from build123d import *

# Parameters (mm, degrees)
SKETCH2_R                                       = 7.5
BOSS_EXTRUDE1_DEPTH                             = 10
CSK_FOR_M4_FLAT_HEAD_MACHINE_SCREW1_D           = 4.3
CSK_FOR_M4_FLAT_HEAD_MACHINE_SCREW1_CSINK_D     = 11.4
CSK_FOR_M4_FLAT_HEAD_MACHINE_SCREW1_CSINK_ANGLE = 90
FILLET1_R                                       = 20
V_GROOVE_CUTOUT_DEPTH                           = 3.6
STANDARD_TAPERED_INSERT_CUTOUT_DEPTH            = 59.209110795
STANDARD_TAPERED_INSERT_CUTOUT_DEPTH_BACK       = 59.209110795
SKETCH13_R                                      = 2.25
TAPER_FOR_INSERTS_SIZE                          = 0.4
TAPER_FOR_INSERTS_SIZE2                         = 1.098990968
MOVE_FACE1_BY                                   = 0.5
MOVE_FACE1_2_BY                                 = 0.5
MOVE_FACE1_3_BY                                 = 0.5
MOVE_FACE1_4_BY                                 = 0.5
MOVE_FACE1_5_BY                                 = 0.5
MOVE_FACE1_6_BY                                 = 0.5
CIRPATTERN2_COUNT                               = 3
FILLET2_R                                       = 3
SKETCH47_R                                      = 1.7
CUT_EXTRUDE1_DEPTH                              = 58.559983963
SKETCH49_W                                      = 15
SKETCH49_H                                      = 10
SKETCH49_W_2                                    = 10
SKETCH49_H_2                                    = 3
BOSS_EXTRUDE2_DEPTH                             = 40
CHAMFER1_SIZE                                   = 2
BOSS_EXTRUDE3_REACH                             = 78.74
SKETCH51_W                                      = 3
SKETCH51_H                                      = 10
BOSS_EXTRUDE4_DEPTH                             = 10
SKETCH48_R                                      = 1.7
CUT_EXTRUDE2_DEPTH                              = 93.266742447
CHAMFER4_SIZE                                   = 2
CHAMFER3_SIZE                                   = 2


with BuildPart() as part:
    # Sketch2 → Boss-Extrude1 (new body)
    with BuildSketch(Plane.XY):
        Polygon((-24.25, 45), (24.25, 45), (24.25, -5.917840259), (35.54293994, -12.437822174), (29.54293994, -22.830127019), (-29.54293994, -22.830127019), (-35.54293994, -12.437822174), (-24.25, -5.917840259), align=None)
        Circle(SKETCH2_R, mode=Mode.SUBTRACT)
    extrude(amount=BOSS_EXTRUDE1_DEPTH)

    # CSK for M4 Flat Head Machine Screw1 (through all)
    with Locations(Plane.XY.offset(10)):
        with Locations((-25.980762114, -15), (0, 30), (25.980762114, -15)):
            CounterSinkHole(CSK_FOR_M4_FLAT_HEAD_MACHINE_SCREW1_D / 2, CSK_FOR_M4_FLAT_HEAD_MACHINE_SCREW1_CSINK_D / 2, counter_sink_angle=CSK_FOR_M4_FLAT_HEAD_MACHINE_SCREW1_CSINK_ANGLE)

    # Fillet1
    fillet1_edges = [part.edges().sort_by_distance(p)[0] for p in [
        (24.25, -5.917840259, 5),
        (-24.25, -5.917840259, 5),
    ]]
    fillet(fillet1_edges, radius=FILLET1_R)

    # Sketch44 → v-groove cutout (cut)
    with BuildSketch(Plane(origin=(0, 0, 0), x_dir=(-1, 0, 0), z_dir=(0, 0, -1))):
        with BuildLine():
            Line((10.392304845, 10), (-10.392304845, 10))
            ThreePointArc((-10.392304845, 10), (-13.856406461, 8), (-13.856406461, 4))
            Line((-13.856406461, 4), (-3.464101615, -14))
            ThreePointArc((-3.464101615, -14), (0, -16), (3.464101615, -14))
            Line((3.464101615, -14), (13.856406461, 4))
            ThreePointArc((13.856406461, 4), (13.856406461, 8), (10.392304845, 10))
        make_face()
    extrude(amount=-V_GROOVE_CUTOUT_DEPTH, mode=Mode.SUBTRACT)

    # Sketch13 → standard tapered insert cutout (cut, two sides: drawn at the far end of the back side and taken through both)
    with BuildSketch(Plane(origin=(0, 0, 0), x_dir=(-1, 0, 0), z_dir=(0, 0, -1)).offset(-STANDARD_TAPERED_INSERT_CUTOUT_DEPTH_BACK)):
        with Locations((-10.392304845, 6)):
            Circle(SKETCH13_R)
        with Locations((10.392304845, 6)):
            Circle(SKETCH13_R)
        with Locations((0, -12)):
            Circle(SKETCH13_R)
    extrude(amount=STANDARD_TAPERED_INSERT_CUTOUT_DEPTH + STANDARD_TAPERED_INSERT_CUTOUT_DEPTH_BACK, mode=Mode.SUBTRACT)

    # taper for inserts
    taper_for_inserts_edges = [part.edges().sort_by_distance(p)[0] for p in [
        (12.642304845, 6, 10),
        (-8.142304845, 6, 10),
        (2.25, -12, 10),
    ]]
    taper_for_inserts_side = [part.faces().sort_by_distance(p)[0] for p in [
        (0, 10.687623267, 10),
    ]]
    chamfer(taper_for_inserts_edges, length=TAPER_FOR_INSERTS_SIZE, length2=TAPER_FOR_INSERTS_SIZE2, reference=taper_for_inserts_side[0])

    # Move Face1: a face moved inward by 0.5
    extrude(part.faces().sort_by_distance((-8.660254038, -5, 1.8))[0], amount=MOVE_FACE1_BY, dir=(-0.866025404, -0.5, 0), mode=Mode.SUBTRACT)

    # Move Face1 2: a curved face moved inward by 0.5
    add(Solid.thicken(part.faces().sort_by_distance((0, -16, 1.8))[0], -MOVE_FACE1_2_BY), mode=Mode.SUBTRACT)

    # Move Face1 3: a face moved inward by 0.5
    extrude(part.faces().sort_by_distance((8.660254038, -5, 1.8))[0], amount=MOVE_FACE1_3_BY, dir=(0.866025404, -0.5, 0), mode=Mode.SUBTRACT)

    # Move Face1 4: a curved face moved inward by 0.5
    add(Solid.thicken(part.faces().sort_by_distance((13.856406461, 8, 1.8))[0], -MOVE_FACE1_4_BY), mode=Mode.SUBTRACT)

    # Move Face1 5: a curved face moved inward by 0.5
    add(Solid.thicken(part.faces().sort_by_distance((-13.856406461, 8, 1.8))[0], -MOVE_FACE1_5_BY), mode=Mode.SUBTRACT)

    # Move Face1 6: a face moved inward by 0.5
    extrude(part.faces().sort_by_distance((0, 10, 1.8))[0], amount=MOVE_FACE1_6_BY, dir=(0, 1, 0), mode=Mode.SUBTRACT)

    # Sketch46 → tool ball cutout (revolve, cut)
    with BuildSketch(Plane(origin=(0, 30, 0), x_dir=(1, 0, 0), z_dir=(0, 1, 0))):
        with BuildLine():
            Line((0, 5.3), (0, -4.7))
            ThreePointArc((0, -4.7), (-5, 0.3), (0, 5.3))
        make_face()
    tool_ball_cutout = revolve(axis=Axis((0, 30, 0), (0, 0, -1)), mode=Mode.SUBTRACT)

    # CirPattern2: tool ball cutout ×3 about axis
    cirpattern2_axis = Axis((0, 0, 0), (0, 0, 1))
    for i in range(1, CIRPATTERN2_COUNT):
        add(tool_ball_cutout.rotate(cirpattern2_axis, i * 360 / CIRPATTERN2_COUNT), mode=Mode.SUBTRACT)

    # Fillet2
    fillet2_edges = [part.edges().sort_by_distance(p)[0] for p in [
        (24.25, 45, 5),
        (-24.25, 45, 5),
        (-29.54293994, -22.830127019, 5),
        (-35.54293994, -12.437822174, 5),
        (29.54293994, -22.830127019, 5),
        (35.54293994, -12.437822174, 5),
    ]]
    fillet(fillet2_edges, radius=FILLET2_R)

    # Sketch47 → Cut-Extrude1 (cut, through all)
    with BuildSketch(Plane(origin=(0, 0, 0), x_dir=(-1, 0, 0), z_dir=(0, 0, -1))):
        with Locations((-17, 27)):
            Circle(SKETCH47_R)
        with Locations((17, 27)):
            Circle(SKETCH47_R)
        with Locations((17, -7)):
            Circle(SKETCH47_R)
        with Locations((-17, -7)):
            Circle(SKETCH47_R)
    extrude(amount=-CUT_EXTRUDE1_DEPTH, mode=Mode.SUBTRACT)

    # Sketch49 → Boss-Extrude2 (add)
    with BuildSketch(Plane(origin=(0, 45, 0), x_dir=(1, 0, 0), z_dir=(0, 1, 0))):
        with Locations((16.75, -5)):
            Rectangle(SKETCH49_W, SKETCH49_H)
        with Locations((16.75, -5)):
            Rectangle(SKETCH49_W_2, SKETCH49_H_2, mode=Mode.SUBTRACT)
    extrude(amount=BOSS_EXTRUDE2_DEPTH)

    # Chamfer1
    chamfer1_edges = [part.edges().sort_by_distance(p)[0] for p in [
        (18.7, -7, 0),
        (-15.3, -7, 0),
        (-15.3, 27, 0),
        (18.7, 27, 0),
    ]]
    chamfer(chamfer1_edges, length=CHAMFER1_SIZE)

    # Sketch51 → Boss-Extrude3 (add, up to next)
    with BuildSketch(Plane.XZ.offset(-45), mode=Mode.PRIVATE) as boss_extrude3_sk1:
        with Locations((22.75, 5)):
            Rectangle(SKETCH51_W, SKETCH51_H)
    boss_extrude3_tool1 = extrude(boss_extrude3_sk1.sketch, amount=BOSS_EXTRUDE3_REACH, mode=Mode.PRIVATE) - part.part
    add(boss_extrude3_tool1.solids().sort_by_distance((22.75, 45, 5))[0])

    # Sketch52 → Boss-Extrude4 (add)
    with BuildSketch(Plane.XY.offset(10)):
        with BuildLine():
            Line((24.25, 45), (31.75, 45))
            Line((31.75, 45), (31.75, -9.983329871))
            ThreePointArc((31.75, -9.983329871), (26.222243623, -3.031088913), (24.25, 5.629165125))
            Line((24.25, 5.629165125), (24.25, 45))
        make_face()
    extrude(amount=-BOSS_EXTRUDE4_DEPTH)

    # Sketch48 → Cut-Extrude2 (cut, through all)
    with BuildSketch(Plane.XY.offset(10)):
        with Locations((0.150338606, 41)):
            Circle(SKETCH48_R)
        with Locations((15.750338606, 41)):
            Circle(SKETCH48_R)
    extrude(amount=-CUT_EXTRUDE2_DEPTH, mode=Mode.SUBTRACT)

    # Chamfer4
    chamfer4_edges = [part.edges().sort_by_distance(p)[0] for p in [
        (-1.549661394, 41, 0),
        (14.050338606, 41, 0),
    ]]
    chamfer(chamfer4_edges, length=CHAMFER4_SIZE)

    # Chamfer3
    chamfer3_edges = [part.edges().sort_by_distance(p)[0] for p in [
        (16.75, 85, 0),
        (9.25, 65, 0),
        (24.25, 65, 0),
    ]]
    chamfer(chamfer3_edges, length=CHAMFER3_SIZE)


solid = part.part
Can you work these out from the model? Positions are in its coordinate system, mm. A direction names the side the tool comes from. Coordinates: 2 decimals unless noted, no trailing zeros. Write each loop counter-clockwise with the first axis right and the second up, starting at its lowest first coordinate (ties: lowest second). Pieces come first, ordered by that corner, then holes.
Q1. Imagine slicing it at A-A, the plane y = 54. List the corners of the cut face in (x, z) for me.
Results found:
outline: (9.25, 2) - (11.25, 0) - (22.25, 0) - (24.25, 2) - (24.25, 10) - (9.25, 10) - close; hole (11.75, 3.5) - (21.75, 3.5) - (21.75, 6.5) - (11.75, 6.5) - close
Q2. If we mould it in two halves opening along Y, with no side actions, what happens to faces 1 (the face through (-24.27, -13.43, 6.62)), 2 (the face through (28, 45, 5)), 3 (the face through (8, 20, 10))? For each: +Y half, -Y half, draft (parallel to the pull), parting line (faces both ways), or undercut.
Results found:
face 1: undercut
face 2: +Y half
face 3: draft
Q3. Imagine slicing it at C-C, the plane x = 0.5. Count the separate pieces of the cut face and the enclosed holes in it, plus the area to 3 significant figures.
Results found:
separate pieces: 5
enclosed holes: 0
area: 348 mm2
Q4. Imagine slicing it at B-B, the plane y = -1.5. List the corners of the cut face in (x, z) for me, plus the area to 3 significant figures.
Results found:
outline: (-25.56, 0) - (-11.26, 0) - (-11.26, 3.6) - (-7.35, 3.6) - (-7.35, 10) - (-25.56, 10) - close; (7.35, 3.6) - (11.26, 3.6) - (11.26, 0) - (31.75, 0) - (31.75, 10) - (7.35, 10) - close
area: 398 mm2
Q5. Please list where these lines run through material, in increasing order: L1, parallel to Y at x = -17, z = 9; L2, parallel to Y at x = 0, z = 6; L3, parallel to X at y = 63.5, z = 4.75.
Results found:
L1: y = -22.83 to -8.7, -5.3 to 25.3, 28.7 to 45
L2: y = -22.83 to -14.25, -9.75 to -7.5, 7.5 to 27.85, 32.15 to 39.31, 42.69 to 45
L3: x = 9.25 to 11.75, 21.75 to 24.25
Q6. For P1, Ø1.5, axis at x = 15.5, z = 4.5, coming from the +Y side; P2, Ø4, axis at y = 69.5, z = 5.5, coming from the +X side; P3, Ø4, axis at y = 15, z = 1.5, coming from the +X side, each with a flat end and sliding along its axis, tell me the tip position at first contact or that it passes through.
Results found:
P1: stops at y = 45
P2: stops at x = 24.25
P3: stops at x = 31.75
Q7. Which directions (+Z, -Z, +X, -X, +Y, -Y) give clear straight access to the entire face, cutting with the end or side of a thin tool? Please do faces 4 (the face through (16.2, -8.5, 5.9)), 5 (the face through (7, 6, 3.6)).
Results found:
face 4: +Z, -Z
face 5: -Z
